```python
from build123d import *

# Parameters (mm, degrees)
BOSS_EXTRUDE1_DEPTH      = 6
SKETCH4_R                = 1.65
CUT_EXTRUDE1_DEPTH       = 7
BOSS_EXTRUDE2_DEPTH      = 2.5
BOSS_EXTRUDE2_DEPTH_BACK = 2.5
FILLET1_R                = 0.1
BOSS_EXTRUDE3_DEPTH      = 3
SKETCH9_R                = 2.75
CUT_EXTRUDE2_DEPTH       = 3
TOLERANCECUT_DEPTH       = 12.0000001
TOLERANCECUT2_DEPTH      = 2.35
TOLERANCECUT2_DEPTH_BACK = 2.35
CUT_EXTRUDE_THIN1_DEPTH  = 10


with BuildPart() as part:
    # Sketch1 → Boss-Extrude1 (new body)
    with BuildSketch(Plane(origin=(0, 0, 0), x_dir=(0, 1, 0), z_dir=(0, 0, 1))):
        with BuildLine():
            Line((66.793011614, 25.63943495), (52.789305216, 20.263915707))
            ThreePointArc((52.789305216, 20.263915707), (42.645904251, 37.130363258), (27.335841873, 49.498371429))
            Line((27.335841873, 49.498371429), (34.587369472, 62.629073903))
            ThreePointArc((34.587369472, 62.629073903), (53.95881545, 46.980136869), (66.793011614, 25.63943495))
        make_face()
    extrude(amount=BOSS_EXTRUDE1_DEPTH)

    # Sketch4 → Cut-Extrude1 (cut, through all)
    with BuildSketch(Plane(origin=(0, 0, 0), x_dir=(0, 1, 0), z_dir=(0, 0, 1))):
        with Locations((41.364521778, 47.584439033)):
            Circle(SKETCH4_R)
        with Locations((53.469432463, 33.41140961)):
            Circle(SKETCH4_R)
    extrude(amount=CUT_EXTRUDE1_DEPTH, mode=Mode.SUBTRACT)

    # Sketch7 → Boss-Extrude2 (add, two sides)
    with BuildSketch(Plane(origin=(0, 0, 0), x_dir=(0, 0, 1), z_dir=(-0.75419408, -0.656651574, 0))) as boss_extrude2_sk:
        with BuildLine():
            Line((6, 41.545), (3, 41.545))
            Line((3, 41.545), (0.5, 44.045))
            Line((0.5, 44.045), (0.5, 44.295))
            Line((0.5, 44.295), (3, 44.295))
            ThreePointArc((3, 44.295), (2.368624388, 50.546249875), (0.5, 56.545))
            Line((0.5, 56.545), (6, 56.545))
            Line((6, 56.545), (6, 44.545))
            Line((6, 44.545), (11, 44.545))
            Line((11, 44.545), (11, 41.545))
            Line((11, 41.545), (6, 41.545))
        make_face()
    extrude(amount=BOSS_EXTRUDE2_DEPTH)
    extrude(boss_extrude2_sk.sketch, amount=-BOSS_EXTRUDE2_DEPTH_BACK)

    # Fillet1
    fillet1_edges = [part.edges().sort_by_distance(p)[0] for p in [
        (-37.130363258, 42.645904251, 0.5),
        (-29.086381475, 33.407026771, 3),
        (-29.250544368, 33.595575291, 6),
    ]]
    fillet(fillet1_edges, radius=FILLET1_R)

    # Sketch8 → Boss-Extrude3 (add)
    with BuildSketch(Plane(origin=(0, 0, 0), x_dir=(0, 1, 0), z_dir=(0, 0, 1))):
        with BuildLine():
            Line((30.796614235, 47.422627264), (28.07341906, 43.229274425))
            ThreePointArc((28.07341906, 43.229274425), (31.734270746, 40.618014295), (35.153605469, 37.69762655))
            Line((35.153605469, 37.69762655), (38.56359727, 41.354395058))
            ThreePointArc((38.56359727, 41.354395058), (34.812578122, 44.558068063), (30.796614235, 47.422627264))
        make_face()
        with BuildLine():
            Line((51.247173818, 23.89694961), (46.715634883, 21.783858301))
            ThreePointArc((46.715634883, 21.783858301), (44.639279438, 25.7725), (42.223192123, 29.564997412))
            Line((42.223192123, 29.564997412), (46.318952344, 32.432879593))
            ThreePointArc((46.318952344, 32.432879593), (48.969406457, 28.2725), (51.247173818, 23.89694961))
        make_face()
    extrude(amount=BOSS_EXTRUDE3_DEPTH)

    # Sketch9 → Cut-Extrude2 (cut)
    with BuildSketch(Plane.XY.offset(6)):
        with Locations((-47.584439033, 41.364521778)):
            Circle(SKETCH9_R)
        with Locations((-33.41140961, 53.469432463)):
            Circle(SKETCH9_R)
    extrude(amount=-CUT_EXTRUDE2_DEPTH, mode=Mode.SUBTRACT)

    # Sketch10 → ToleranceCut (cut, through all)
    with BuildSketch(Plane(origin=(0, 0, 0), x_dir=(0, 1, 0), z_dir=(0, 0, 1))):
        with BuildLine():
            Line((38.453894214, 41.456694812), (35.14605375, 37.9094702))
            ThreePointArc((35.14605375, 37.9094702), (31.826619967, 40.736215908), (28.280796974, 43.273196641))
            Line((28.280796974, 43.273196641), (30.92241482, 47.340931409))
            Line((30.92241482, 47.340931409), (30.67081365, 47.50432312))
            Line((30.67081365, 47.50432312), (27.865803402, 43.184986115))
            ThreePointArc((27.865803402, 43.184986115), (31.641921524, 40.499812682), (35.160859486, 37.485463652))
            Line((35.160859486, 37.485463652), (38.673300325, 41.252095304))
            Line((38.673300325, 41.252095304), (38.453894214, 41.456694812))
        make_face()
        with BuildLine():
            Line((46.232915879, 32.5557524), (42.014103544, 29.601708201))
            ThreePointArc((42.014103544, 29.601708201), (44.509375628, 25.6975), (46.642883069, 21.584426886))
            Line((46.642883069, 21.584426886), (51.310566557, 23.761003442))
            Line((51.310566557, 23.761003442), (51.183781079, 24.032895778))
            Line((51.183781079, 24.032895778), (46.787991078, 21.983105237))
            ThreePointArc((46.787991078, 21.983105237), (44.769183249, 25.8475), (42.431923129, 29.528036247))
            Line((42.431923129, 29.528036247), (46.40498881, 32.310006787))
            Line((46.40498881, 32.310006787), (46.232915879, 32.5557524))
        make_face()
        Polygon((44.147333984, 35.321699097), (32.876124251, 25.508233558), (33.073119723, 25.281975334), (44.344329456, 35.095440873), align=None)
        Polygon((40.817854097, 39.052425533), (29.59286638, 29.279203958), (29.789861852, 29.052945734), (41.014849569, 38.826167309), align=None)
    extrude(amount=TOLERANCECUT_DEPTH, mode=Mode.SUBTRACT)

    # Sketch16 → ToleranceCut2 (cut, two sides)
    with BuildSketch(Plane(origin=(0, 0, 0), x_dir=(0, 0, 1), z_dir=(-0.75419408, -0.656651574, 0))) as tolerancecut2_sk:
        with BuildLine():
            Line((5.85, 56.545), (5.85, 44.395))
            Line((5.85, 44.395), (10.85, 44.395))
            Line((10.85, 44.395), (10.85, 41.695))
            Line((10.85, 41.695), (6, 41.695))
            Line((6, 41.695), (3.062132034, 41.695))
            Line((3.062132034, 41.695), (0.65, 44.107132034))
            Line((0.65, 44.107132034), (0.65, 44.145))
            Line((0.65, 44.145), (3.14964186, 44.145))
            ThreePointArc((3.14964186, 44.145), (2.530504313, 50.50274046), (0.638004798, 56.603776489))
            Line((0.638004798, 56.603776489), (0.361995202, 56.486223511))
            ThreePointArc((0.361995202, 56.486223511), (2.206568162, 50.589723315), (2.849638407, 44.445))
            Line((2.849638407, 44.445), (0.35, 44.445))
            Line((0.35, 44.445), (0.35, 43.982867966))
            Line((0.35, 43.982867966), (2.937867966, 41.395))
            Line((2.937867966, 41.395), (6, 41.395))
            Line((6, 41.395), (11.15, 41.395))
            Line((11.15, 41.395), (11.15, 44.695))
            Line((11.15, 44.695), (6.15, 44.695))
            Line((6.15, 44.695), (6.15, 56.545))
            Line((6.15, 56.545), (5.85, 56.545))
        make_face()
    extrude(amount=TOLERANCECUT2_DEPTH, mode=Mode.SUBTRACT)
    extrude(tolerancecut2_sk.sketch, amount=-TOLERANCECUT2_DEPTH_BACK, mode=Mode.SUBTRACT)

    # Sketch17 → Cut-Extrude-Thin1 (cut)
    with BuildSketch(Plane(origin=(0, 0, 0), x_dir=(0, 1, 0), z_dir=(0, 0, 1))):
        with BuildLine():
            ThreePointArc((51.047913396, 23.969100589), (51.912040519, 22.035137719), (52.70292998, 20.070087611))
            Line((52.70292998, 20.070087611), (66.846766806, 25.499397886))
            Line((66.846766806, 25.499397886), (66.739256421, 25.779472014))
            Line((66.739256421, 25.779472014), (52.875494708, 20.457672502))
            ThreePointArc((52.875494708, 20.457672502), (52.129243688, 22.290721328), (51.319468445, 24.096606884))
            Line((51.319468445, 24.096606884), (51.047913396, 23.969100589))
        make_face()
        with BuildLine():
            ThreePointArc((31.004335746, 47.466347973), (29.290610597, 48.542591153), (27.539568245, 49.556989475))
            Line((27.539568245, 49.556989475), (34.718676497, 62.556558627))
            Line((34.718676497, 62.556558627), (34.456062447, 62.701589179))
            Line((34.456062447, 62.701589179), (27.131923134, 49.439405054))
            ThreePointArc((27.131923134, 49.439405054), (29.007426552, 48.362849687), (30.840277175, 47.215181126))
            Line((30.840277175, 47.215181126), (31.004335746, 47.466347973))
        make_face()
        with BuildLine():
            ThreePointArc((38.351817991, 41.346648013), (39.675403143, 40.078293758), (40.957064996, 38.767590486))
            Line((40.957064996, 38.767590486), (41.174940656, 38.973818992))
            ThreePointArc((41.174940656, 38.973818992), (39.88646086, 40.291494696), (38.55583475, 41.566596103))
            Line((38.55583475, 41.566596103), (38.351817991, 41.346648013))
        make_face()
        with BuildLine():
            ThreePointArc((44.030208622, 35.227988641), (45.178364811, 33.742937157), (46.276455334, 32.220492496))
            Line((46.276455334, 32.220492496), (46.522656602, 32.391912844))
            ThreePointArc((46.522656602, 32.391912844), (45.418723987, 33.922457258), (44.264459346, 35.415409553))
            Line((44.264459346, 35.415409553), (44.030208622, 35.227988641))
        make_face()
    extrude(amount=CUT_EXTRUDE_THIN1_DEPTH, mode=Mode.SUBTRACT)


solid = part.part
```
The model under review builds one solid part; all positions refer to its coordinate system, in mm. A direction names the side the tool comes from. Round coordinates to 2 decimals unless told otherwise and drop trailing zeros. Loops run counter-clockwise (first coordinate to the right, second up) from the corner with the lowest first, then second, coordinate; pieces in that order, holes last.
1) The part is to be moulded in two halves that separate along Y. For faces 6 (the face through (-27, 47, 3)), 7 (the face through (-47.24, 53.73, 2.96)), 8 (the face through (-56, 31.1, 3)), say which applies: pulls with the +Y half, pulls with the -Y half, needs draft (parallel to the pull), parting line crosses it, or undercut.
Values follow:
face 6: undercut
face 7: pulls with the +Y half
face 8: pulls with the -Y half
2) Consider section C-C on x = -58.5. State the section outline as (y, z) points, then the cut area to 3 significant figures.
Values follow:
outline: (32.48, 0) - (41.19, 0) - (41.19, 6) - (32.48, 6) - close
area: 52.3 mm2
3) Consider section B-B on y = 54. State the section outline as (x, z) points, then the cut area to 3 significant figures.
Values follow:
outline: (-46.93, 0) - (-34.97, 0) - (-34.97, 3) - (-36.11, 3) - (-36.11, 6) - (-46.93, 6) - close; (-31.85, 0) - (-20.89, 0) - (-20.89, 6) - (-30.71, 6) - (-30.71, 3) - (-31.85, 3) - close
area: 131 mm2
4) Consider section D-D on z = 7.25. State the section outline as (x, y) points, then the cut area to 3 significant figures.
Values follow:
outline: (-30.92, 31.94) - (-29.15, 29.9) - (-25.61, 32.99) - (-27.38, 35.03) - close
area: 12.7 mm2
5) Consider section A-A on z = 2.5. Give the number of separate pieces and of enclosed holes in the cut face, then the cut area to 3 significant figures.
Values follow:
separate pieces: 2
enclosed holes: 2
area: 773 mm2
6) Wall thickness on line 1 along Z through (x, y) = (-43.5, 43.5); line 2 along X through (y, z) = (43, 4.75); line 3 along X through (y, z) = (30.5, 4.75): over which ranges is each line inside the solid? List them lowest first.
Values follow:
line 1: z = 0 to 6
line 2: x = -57.18 to -49.8, -45.37 to -34.32
line 3: x = -54.92 to -47.79, -29.67 to -28.47
7) Tool access review of faces 1 (the face through (-43, 33, 3)), 2 (the face through (-33.901, 45.435, 2.958)), 3 (the face through (-22.27, 52.14, 2.96)), 4 (the face through (-48.53, 29.31, 2.96)), 5 (the face through (-33.769, 56.196, 4.521)): name each direction out of +Z, -Z, +X, -X, +Y, -Y from which nothing blocks a thin tool from reaching the whole face with its end or side.
Values follow:
face 1: +Z, -Y
face 2: +Z, -Z
face 3: +Z, -Z, +X
face 4: +Z, -Z, -Y
face 5: +Z
8) Clearance check with flat-ended pins moving along their axes: P1, Ø5, axis at x = -43.5, z = 1.5, coming from the +Y side; P2, Ø19.5, axis at x = -44, y = 46, coming from the +Z side; P3, Ø6, axis at x = -36.5, z = 1.5, coming from the -Y side; P4, Ø2, axis at y = 50.5, z = 8.5, coming from the -X side. State where each tip first meets the part, or that it passes through.
Values follow:
P1: stops at y = 58.63
P2: stops at z = 6
P3: stops at y = 33.35
P4: passes through
